Design review of the part shown in the three views and the two pictorial views. Dimensions are in mm from the part's minimum x, y and z. Round coordinates to 2 decimals unless told otherwise and drop trailing zeros. Loops run counter-clockwise (first coordinate to the right, second up) from the corner with the lowest first, then second, coordinate; pieces in that order, holes last. Notation, with made-up numbers: M 33.5,14 L 85.5,14 A33 cw 85.5,50 Z; hole C 20.5,9 d6. An arc over 180 degrees is marked long. Return JSON: item names as keys, results as strings. Group by question number.
Q1. Clearance check with flat-ended pins moving along their axes: pin 1 Ø2 at (y, z) = (14, 13.5) entering from -X; pin 2 Ø11 at (y, z) = (10, 10) entering from +X. State where each tip first meets the part, or that it passes through.
Q2. To check wall thickness, follow line 1 along Z through (x, y) = (2.2, 10); line 2 along Z through (x, y) = (4.75, 10); line 3 along X through (y, z) = (5.75, 17.25). State the ranges of each line that lie inside material, in increasing order.
Q3. Consider section A-A (y = 10). State the section outline as (x, z) points.
Q4. Draft analysis for pull direction Z (two halves, no side actions). For the marked faces 1, 2, 3 and 4, state which applies: pulls with the +Z half, pulls with the -Z half, needs draft (parallel to the pull), parting line crosses it, or undercut.
Q5. Consider section D-D (x = 2.9). State the section outline as (y, z) points.
Q6. Consider section C-C (z = 2.75). State the section outline as (x, y) points.
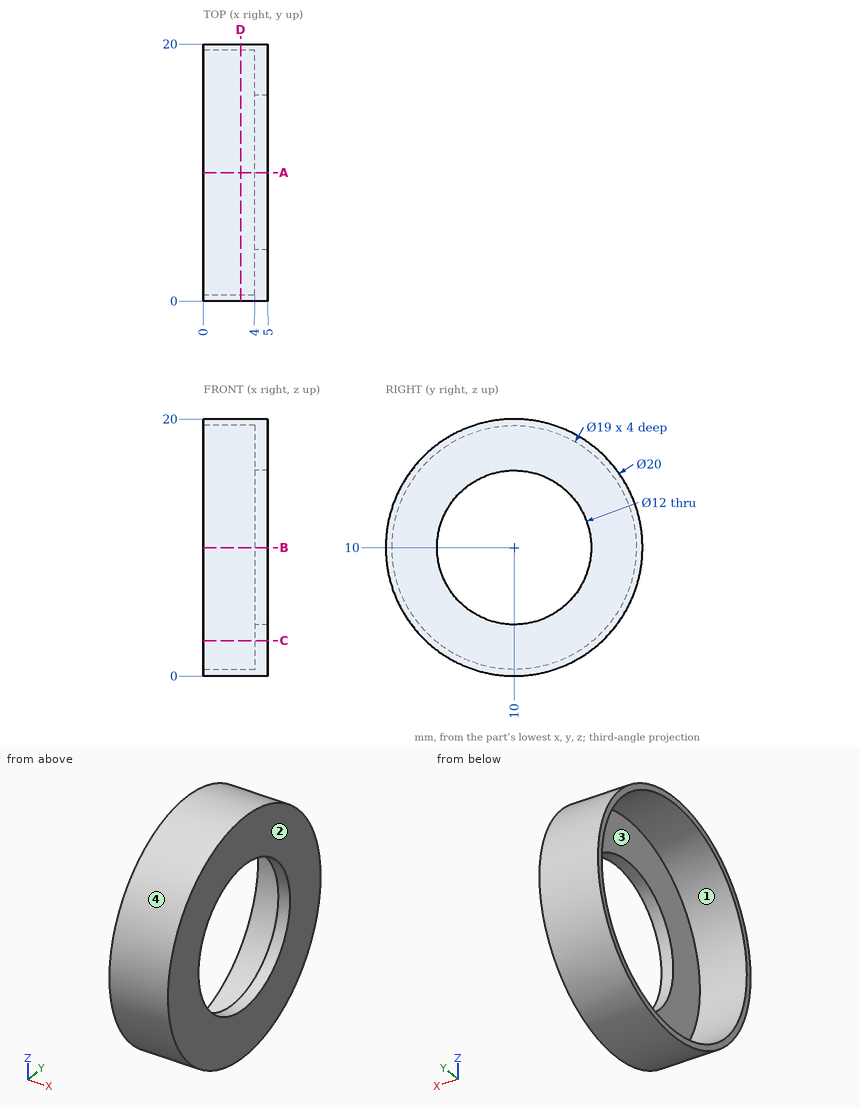
Values:
{
 "1": {"pin 1": "stops at x = 4", "pin 2": "passes through"},
 "2": {"line 1": "z = 0 to 0.5, 19.5 to 20", "line 2": "z = 0 to 4, 16 to 20", "line 3": "x = 4 to 5"},
 "3": {"outline": "M 0,0 L 5,0 L 5,4 L 4,4 L 4,0.5 L 0,0.5 Z; M 0,19.5 L 4,19.5 L 4,16 L 5,16 L 5,20 L 0,20 Z"},
 "4": {"face 1": "undercut", "face 2": "needs draft", "face 3": "undercut", "face 4": "parting line crosses it"},
 "5": {"outline": "C 10,10 d20; hole C 10,10 d19"},
 "6": {"outline": "M 0,3.11 L 5,3.11 L 5,16.89 L 0,16.89 L 0,16.14 L 4,16.14 L 4,3.86 L 0,3.86 Z"}
}
